Input: part model. Units: mm. Frame: model coordinates. Face numbers are marked on the shaded views. A direction names the side the tool comes from. Coordinates: 2 decimals unless noted, no trailing zeros. Write each loop counter-clockwise with the first axis right and the second up, starting at its lowest first coordinate (ties: lowest second). Pieces come first, ordered by that corner, then holes. Notation, with made-up numbers: M 61,58 L 89,58 A24 ccw 89,91 Z; hole C 56.25,10.5 d3. An arc over 180 degrees is marked long. Use CSV: the item, a comma, the result in double quotes.
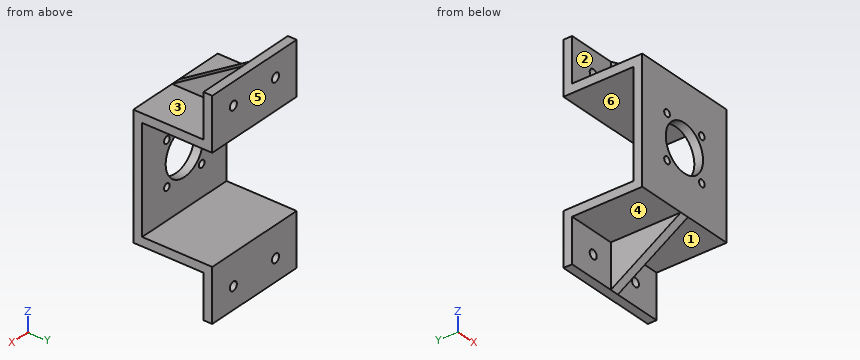
Autodesk Inventor part; units mm, degrees
ref_plane "Work Plane3" through (0, -5, 35) normal (1, 0, 0) x (0, 0, -1)
ref_plane "YZ Plane" through (0, 0, 0) normal (1, 0, 0) x (0, 1, 0)
ref_plane "XZ Plane" through (0, 0, 0) normal (0, 1, 0) x (-1, 0, 0)
sketch "Sketch1" plane through (0, 0, 0) normal (0, 1, 0) x (-1, 0, 0)
  circle A0 centre (0, 0) radius 13.25
  line L0 (0, 0) -> (12.3744, 12.3744) construction
  line L1 (0, 0) -> (17.5, 0) construction
  line L2 (0, 0) -> (-12.3744, -12.3744) construction
  line L3 (0, 0) -> (17.5, 0) construction
  circle A1 centre (-12.3744, -12.3744) radius 2
  circle A2 centre (12.3744, 12.3744) radius 2
  circle A3 centre (12.3744, -12.3744) radius 2
  circle A4 centre (-12.3744, 12.3744) radius 2
  circle A5 centre (0, 0) radius 17.5 construction
  line L4 (30, 30) -> (-30, 30)
  line L5 (-30, 30) -> (-30, -30)
  line L6 (-30, -30) -> (30, -30)
  line L7 (30, -30) -> (30, 30)
  line L8 (30, 30) -> (-30, -30) construction
  line L9 (-30, 30) -> (30, -30) construction
  line L10 (30, -30) -> (-30, -30)
  line L11 (-30, -30) -> (-30, -35)
  line L12 (-30, -35) -> (30, -35)
  line L13 (30, -35) -> (30, -30)
  line L14 (30, 30) -> (-30, 30)
  line L15 (-30, 30) -> (-30, 35)
  line L16 (-30, 35) -> (30, 35)
  line L17 (30, 35) -> (30, 30)
  dimension "d0" = 26.5
  dimension "d1" = 17.5
  dimension "d2" = 45
  dimension "d3" = 17.5
  dimension "d4" = 135
  dimension "d5" = 4
  dimension "d6" = 4
  dimension "d7" = 60
  dimension "d9" = 5
  dimension "d10" = 5
extrude "Extrusion1" add sketch "Sketch1" against normal blind 5
extrude "Extrusion2" add sketch "Sketch1" along normal blind 35 contours L4 L15 L16 L17 | L13 L12 L11 L6
sketch "Sketch4" plane through (-30, 35, 30) normal (0, 1, 0) x (1, 0, 0)
  line L0 (0, 60) -> (0, 0) construction
  line L1 (0, -30) -> (60, -30) construction
  line L2 (30, -17.5) -> (45, -17.5) construction
  line L3 (60, -5) -> (60, -30) construction
  line L4 (30, -17.5) -> (15, -17.5) construction
  circle A0 centre (45, -17.5) radius 2.5
  circle A1 centre (15, -17.5) radius 2.5
  line L5 (60, 0) -> (0, 0)
  line L6 (0, 0) -> (0, -30)
  line L7 (60, -30) -> (0, -30)
  line L8 (60, 0) -> (60, -30)
  line L9 (0, 60) -> (60, 60)
  line L10 (60, 60) -> (60, 90)
  line L11 (60, 90) -> (0, 90)
  line L12 (0, 90) -> (0, 60)
  line L13 (60, 0) -> (0, 0)
  line L14 (0, 0) -> (60, 0)
  line L15 (60, -5) -> (0, -5)
  line L16 (60, -30) -> (0, -30)
  line L17 (0, -30) -> (0, -5)
  line L18 (0, -5) -> (60, -5)
  line L19 (60, -5) -> (60, -30)
  line L20 (60, -30) -> (0, -5) construction
  line L21 (30, -17.5) -> (30, -30) construction
  line L22 (30, 77.5) -> (45, 77.5) construction
  line L23 (30, 77.5) -> (15, 77.5) construction
  circle A2 centre (45, 77.5) radius 2.5
  circle A3 centre (15, 77.5) radius 2.5
  line L24 (60, 65) -> (0, 65)
  line L25 (0, 65) -> (0, 90)
  line L26 (0, 90) -> (60, 90)
  line L27 (60, 90) -> (60, 65)
  line L28 (60, 65) -> (0, 90) construction
  line L29 (30, 77.5) -> (30, 65) construction
  point P0 (30, 30)
  dimension "d19" = 15
  dimension "d20" = 5
  dimension "d28" = 15
  dimension "d29" = 5
extrude "Extrusion4" add sketch "Sketch4" along normal blind 5
ref_plane "Work Plane3" through (0, -5, 35) normal (1, 0, 0) x (0, 0, -1)
sketch "Sketch5" plane through (0, -5, 35) normal (1, 0, 0) x (0, 0, -1)
  line L0 (0, 40) -> (0, 0)
  line L1 (0, 0) -> (0, 40)
  line L2 (0, 40) -> (-25, 40)
  line L3 (-25, 45) -> (5, 45)
  line L4 (-25, 40) -> (0, 0)
  line L5 (0, 0) -> (70, 0)
  line L6 (70, 0) -> (70, 40)
  line L7 (70, 0) -> (70, 40)
  line L8 (95, 40) -> (70, 40)
  line L9 (70, 40) -> (95, 40)
  line L10 (95, 40) -> (70, 0)
  point P0 (35, 5)
extrude "Extrusion5" add sketch "Sketch5" along normal mid plane 5
properties part number "Base_Motor_Mount"
1. Contact query for flat-ended pins moving along their axis: pin 1 Ø12.5 at (y, z) = (22.5, -51.5) entering from -X; pin 2 Ø5 at (y, z) = (3.5, -26.5) entering from -X; pin 3 Ø4 at (x, z) = (-14, -9.5) entering from +Y; pin 4 Ø12.5 at (x, z) = (19, -44.5) entering from -Y. Output: stop coordinate, or through.
Resolved:
pin 1,"stops at x = -2.5"
pin 2,"passes through"
pin 3,"stops at y = 0"
pin 4,"stops at y = 35"
2. Material intervals for line 1 (Z direction, x = -15, y = 36); line 2 (Z direction, x = -18, y = 14.5); line 3 (X direction, y = 36.25, z = -47.5), sorted ascending. Write a range as [from, to].
Resolved:
line 1,"z = [-60, -50], [-45, -30], [30, 45], [50, 60]"
line 2,"z = [-35, -30], [30, 35]"
line 3,"x = [-30, -17.5], [-12.5, 12.5], [17.5, 30]"
3. Section C-C (x = 0). Return loops of the section in (y, z), then the cut area to 3 significant figures.
Resolved:
outline,"M -5,-35 L 35,-60 L 40,-60 L 40,-30 L 0,-30 L 0,-13.25 L -5,-13.25 Z; M -5,13.25 L 0,13.25 L 0,30 L 40,30 L 40,60 L 35,60 L -5,35 Z"
area,"1,870 mm^2"
4. Section A-A (y = 19). Return loops of the section in (x, z).
Resolved:
outline,"M -30,-35 L -2.5,-35 L -2.5,-50 L 2.5,-50 L 2.5,-35 L 30,-35 L 30,-30 L -30,-30 Z; M -30,30 L 30,30 L 30,35 L 2.5,35 L 2.5,50 L -2.5,50 L -2.5,35 L -30,35 Z"
5. Section D-D (z = 47.5). Return loops of the section in (x, y).
Resolved:
outline,"M -30,35 L -17.5,35 L -17.5,40 L -30,40 Z; M -12.5,35 L -2.5,35 L -2.5,15 L 2.5,15 L 2.5,35 L 12.5,35 L 12.5,40 L -12.5,40 Z; M 17.5,35 L 30,35 L 30,40 L 17.5,40 Z"
6. Mould query, pull axis Z, two halves, no side actions, for the marked faces 4, 5 and 6. Classes: pulls with the +Z half, pulls with the -Z half, needs draft (parallel to the pull), parting line crosses it, or undercut.
Resolved:
face 4,"pulls with the -Z half"
face 5,"needs draft"
face 6,"undercut"
7. Section B-B (z = 0). Return loops of the section in (x, y).
Resolved:
outline,"M -30,-5 L -13.25,-5 L -13.25,0 L -30,0 Z; M 13.25,-5 L 30,-5 L 30,0 L 13.25,0 Z"
8. Access query for the marked faces 1, 2 and 3. Directions: +Z, -Z, +X, -X, +Y, -Y. A direction counts if a zero-diameter tool reaches every point of the face in a straight line with its end or side. Return the directions, or none.
Resolved:
face 1,"-Z, +X, -Y"
face 2,"+Z, -X, -Y"
face 3,"+Z, +X, -Y"
